Can you work these out from the model? Positions are in its coordinate system, mm. A direction names the side the tool comes from. Round coordinates to 2 decimals unless told otherwise and drop trailing zeros. Order: outer loops, then holes, each group sorted by start corner. A loop starts at its lowest first (then second) coordinate and runs counter-clockwise, first axis right, second up. Notation, with made-up numbers: M 75,41.25 L 109,41.25 A34 ccw 109,72.25 Z; hole C 72,2 d10. An arc over 180 degrees is marked long. Answer as a JSON object with one key per item and string values. Group by question number.
Solid Edge part; units mm, degrees
sketch "Sketch1" plane through (0, 0, 0) normal (0, 0, 1) x (1, 0, 0)
  circle A0 centre (0, 0) radius 3.5
extrude "Protrusion1" add sketch "Sketch1" along normal blind 3.8
sketch "Sketch2" plane through (0, 0, 3.8) normal (0, 0, 1) x (1, 0, 0)
  circle A0 centre (0, 0) radius 2.35
extrude "Extrusionsausschnitt_1" cut sketch "Sketch2" against normal blind 1
sketch "Sketch3" plane through (0, 0, 2.8) normal (0, 0, 1) x (1, 0, 0)
  circle A0 centre (0, 0) radius 1.25
extrude "Cutout1" cut sketch "Sketch3" against normal through all
sketch "Sketch4" plane through (0, 0, 0) normal (0, 0, -1) x (1, 0, 0)
  circle A0 centre (0, 0) radius 2.35
extrude "Extrusionsausschnitt_3" cut sketch "Sketch4" against normal blind 2
sketch "Sketch5" plane through (0, 0, 3.8) normal (0, 0, 1) x (1, 0, 0)
  line L0 (-1.95, 2.9065) -> (-1.95, 6.35)
  arc A0 (-1.95, 6.35) -> (1.95, 6.35) centre (0, 6.35) cw
  line L1 (1.95, 6.35) -> (1.95, 3.4)
  line L2 (1.95, 3.4) -> (16.9, 1.8)
  arc A1 (16.9, 1.8) -> (16.9, -1.8) centre (16.6875, 0) cw
  line L3 (16.9, -1.8) -> (1.95, -3.4)
  line L4 (1.95, -3.4) -> (1.95, -6.35)
  arc A2 (-1.95, -6.35) -> (1.95, -6.35) centre (0, -6.35) ccw
  line L5 (-1.95, -2.9065) -> (-1.95, -6.35)
  line L6 (-1.95, -2.9065) -> (-14.5, -1.9)
  arc A3 (-14.5, 1.9) -> (-14.5, -1.9) centre (-14.0467, 0) ccw
  line L7 (-1.95, 2.9065) -> (-14.5, 1.9)
  circle A4 centre (0, 0) radius 2.901
extrude "Extrusionsausprägung_2" add sketch "Sketch5" against normal blind 1.4
sketch "Sketch6" plane through (0, 0, 0) normal (0, 0, 1) x (1, 0, 0)
  circle A0 centre (0, 4.4) radius 0.6
  circle A1 centre (0, 6.2) radius 0.6
  circle A2 centre (0, -6.2) radius 0.6
  circle A3 centre (0, -4.4) radius 0.6
  circle A4 centre (-4.55, 0) radius 0.6
  circle A5 centre (-6.45, 0) radius 0.6
  circle A6 centre (-8.35, 0) radius 0.6
  circle A7 centre (-10.25, 0) radius 0.6
  circle A8 centre (-14.05, 0) radius 0.6
  circle A9 centre (-12.15, 0) radius 0.6
  circle A10 centre (5.05, 0) radius 0.6
  circle A11 centre (6.95, 0) radius 0.6
  circle A12 centre (8.85, 0) radius 0.6
  circle A13 centre (12.65, 0) radius 0.6
  circle A14 centre (14.55, 0) radius 0.6
  circle A15 centre (10.75, 0) radius 0.6
  circle A16 centre (16.45, 0) radius 0.6
extrude "Cutout2" cut sketch "Sketch6" along normal through all
1) If we section it at B-B on x = 12.65: Write out the boundary of the cut face in (y, z).
2) We'd pull the mould along Y, two halves only. Please class faces 4 (the face through (0, -8.3, 3.1)), 5 (the face through (1, -1, 2.8)), 6 (the face through (9.32, 2.61, 3.11)): +Y half, -Y half, draft (parallel to the pull), parting line (faces both ways), or undercut.
3) I need wall thicknesses on line 1 along Z through (x, y) = (-10, -1.25); line 2 along Y through (x, z) = (-1, 3.4); line 3 along Y through (x, z) = (5.05, 2.7). Which ranges of each line are inside material? Lowest first, please.
4) Which directions (+Z, -Z, +X, -X, +Y, -Y) give clear straight access to the entire face, cutting with the end or side of a thin tool? Please do faces 1 (the face through (3.233, 1.341, 1.183)), 2 (the face through (-8.14, -2.41, 3.11)), 3 (the face through (1.95, -5, 3)).
5) If we section it at D-D on z = 0.8: Write out the boundary of the cut face in (x, y).
6) For pin 1 (1.1 mm diameter, centred on x = 14.55, y = 0, fed in from -Z); pin 2 (5.5 mm diameter, centred on x = 0, y = 0, fed in from +Z); pin 3 (1.1 mm diameter, centred on y = -5, z = 3.5, fed in from +X); pin 4 (3 mm diameter, centred on x = 0, y = 0, fed in from -Z), each with a flat end and sliding along its axis, tell me the tip position at first contact or that it passes through.
7) If we section it at A-A on y = -4.4: Write out the boundary of the cut face in (x, z), plus the area to 3 significant figures.
8) If we section it at C-C on y = 0: Count the separate pieces of the cut face and the enclosed holes in it, plus the area to 3 significant figures.
Findings:
{
 "1": {"outline": "M -2.25,2.4 L -0.6,2.4 L -0.6,3.8 L -2.25,3.8 Z; M 0.6,2.4 L 2.25,2.4 L 2.25,3.8 L 0.6,3.8 Z"},
 "2": {"face 4": "-Y half", "face 5": "undercut", "face 6": "+Y half"},
 "3": {"line 1": "z = 2.4 to 3.8", "line 2": "y = -8.02 to -2.13, 2.13 to 8.02", "line 3": "y = -3.07 to -0.6, 0.6 to 3.07"},
 "4": {"face 1": "-Z", "face 2": "+Z, -Z, -X, -Y", "face 3": "+Z, -Z, +X, -Y"},
 "5": {"outline": "C 0,0 d7; hole C 0,0 d4.7"},
 "6": {"pin 1": "passes through", "pin 2": "stops at z = 3.8", "pin 3": "stops at x = 1.95", "pin 4": "stops at z = 2"},
 "7": {"outline": "M -1.95,2.4 L -0.6,2.4 L -0.6,3.8 L -1.95,3.8 Z; M 0.6,2.4 L 1.95,2.4 L 1.95,3.8 L 0.6,3.8 Z", "area": "3.78 mm^2"},
 "8": {"separate pieces": "15", "enclosed holes": "0", "area": "27.2 mm^2"}
}
